from build123d import *

# Parameters (mm, degrees)
F1_DEPTH = 12.7
F2_R     = 1.27


with BuildPart() as f1:
    # F0 (on Top) → F1 (new body)
    with BuildSketch(Plane.XY):
        with BuildLine():
            ThreePointArc((-11.2866647297, 31.0098564859), (0, 33), (11.2866647297, 31.0098564859))
            Line((11.2866647297, 31.0098564859), (11.7129790451, 32.1811454409))
            ThreePointArc((11.7129790451, 32.1811454409), (11.6604357653, 33.1734751566), (10.9094104776, 33.8241978919))
            ThreePointArc((10.9094104776, 33.8241978919), (7.8564465257, 34.6607537135), (4.7411554622, 35.2223373001))
            ThreePointArc((4.7411554622, 35.2223373001), (3.167898391, 36.0676691962), (2.54, 37.7396343385))
            Line((2.54, 37.7396343385), (2.54, 39.2591184658))
            Line((2.54, 39.2591184658), (6.35, 39.2591184658))
            ThreePointArc((6.35, 39.2591184658), (7.2480256121, 39.6310928537), (7.62, 40.5291184658))
            Line((7.62, 40.5291184658), (7.62, 42.4341184658))
            Line((7.62, 42.4341184658), (2.54, 42.4341184658))
            Line((2.54, 42.4341184658), (2.54, 44.9741184658))
            Line((2.54, 44.9741184658), (4.318, 44.9741184658))
            ThreePointArc((4.318, 44.9741184658), (5.2160256121, 45.3460928537), (5.588, 46.2441184658))
            Line((5.588, 46.2441184658), (5.588, 46.5616184658))
            Line((5.588, 46.5616184658), (2.9195765878, 49.6191869589))
            ThreePointArc((2.9195765878, 49.6191869589), (2.488257012, 49.9402838921), (1.9627272727, 50.0541184658))
            Line((1.9627272727, 50.0541184658), (0, 50.0541184658))
            Line((0, 50.0541184658), (-1.9627272727, 50.0541184658))
            ThreePointArc((-1.9627272727, 50.0541184658), (-2.488257012, 49.9402838921), (-2.9195765878, 49.6191869589))
            Line((-2.9195765878, 49.6191869589), (-5.588, 46.5616184658))
            Line((-5.588, 46.5616184658), (-5.588, 46.2441184658))
            ThreePointArc((-5.588, 46.2441184658), (-5.2160256121, 45.3460928537), (-4.318, 44.9741184658))
            Line((-4.318, 44.9741184658), (-2.54, 44.9741184658))
            Line((-2.54, 44.9741184658), (-2.54, 42.4341184658))
            Line((-2.54, 42.4341184658), (-7.62, 42.4341184658))
            Line((-7.62, 42.4341184658), (-7.62, 40.5291184658))
            ThreePointArc((-7.62, 40.5291184658), (-7.2480256121, 39.6310928537), (-6.35, 39.2591184658))
            Line((-6.35, 39.2591184658), (-2.54, 39.2591184658))
            Line((-2.54, 39.2591184658), (-2.54, 37.7396343385))
            ThreePointArc((-2.54, 37.7396343385), (-3.167898391, 36.0676691962), (-4.7411554622, 35.2223373001))
            ThreePointArc((-4.7411554622, 35.2223373001), (-7.8564465257, 34.6607537135), (-10.9094104776, 33.8241978919))
            ThreePointArc((-10.9094104776, 33.8241978919), (-11.6604357653, 33.1734751566), (-11.7129790451, 32.1811454409))
            Line((-11.7129790451, 32.1811454409), (-11.2866647297, 31.0098564859))
        make_face()
    extrude(amount=F1_DEPTH)

    # F2
    f2_edges = [f1.edges().sort_by_distance(p)[0] for p in [
        (3.167898, 36.067669, 12.7),
        (-7.856447, 34.660754, 12.7),
        (-5.08, 42.434118, 12.7),
        (5.08, 42.434118, 12.7),
        (4.253788, 48.090403, 12.7),
    ]]
    fillet(f2_edges, radius=F2_R)


solid = f1.part
CAD build for the part. Positions are in the model's coordinates, mm. A direction names the side the tool comes from. Round coordinates to 2 decimals unless told otherwise and drop trailing zeros. Write each loop counter-clockwise with the first axis right and the second up, starting at its lowest first coordinate (ties: lowest second). Pieces come first, ordered by that corner, then holes. Notation, with made-up numbers: M -22.5,-19.5 L 19.5,-19.5 A23 ccw 19.5,13.5 Z; hole C 4.25,-14.75 d7. An arc over 180 degrees is marked long. Use a Markdown table: item, result. Add a question column.
1. Pull direction Y, two halves, no side cores. Call faces 1 (the face through (-2.481, 49.943, 5.635)), 2 (the face through (7.238, 39.621, 6.261)), 3 (the face through (0, 40, 12.7)), 4 (the face through (11.16, 31.72, 12.32)): released by +Y, released by -Y, zero draft, split by the parting line, or undercut.
2. 3-axis set-ups, long thin cutter, end or side, ignore diameter. For faces 5 (the face through (5, 42.434, 6)), 6 (the face through (7.62, 41, 6)), 7 (the face through (-7.81, 34.67, 5.63)): which of +Z, -Z, +X, -X, +Y, -Y reach the whole face in a straight line?
3. Slice it at B-B on y = 42. Give the cut face in (x, z), then the cut area to 3 significant figures.
4. Drill centre lines: probe 1 along X at (y, z) = (46.25, 9.5); probe 2 along Y at (x, z) = (-5, 7); probe 3 along X at (y, z) = (44, 10.5). Where is each one in solid material? Low to high.
5. Slice it at C-C on x = -3.75. Give the number of separate pieces and of enclosed holes in the cut face, then the cut area to 3 significant figures.
6. Flat gauge pins, fed straight in: P1, Ø1.9, axis at y = 43.5, z = 7, coming from the -X side; P2, Ø1.5, axis at x = 4.5, z = 3.5, coming from the +Y side; P3, Ø2, axis at x = -3, z = 4, coming from the -Y side. Where does each tip first touch, or does it go through?
Reply:
| question | item | result |
|---|---|---|
| 1 | face 1 | released by +Y |
| 1 | face 2 | undercut |
| 1 | face 3 | zero draft |
| 1 | face 4 | released by -Y |
| 2 | face 5 | +Z, -Z, +X |
| 2 | face 6 | +Z, -Z, +X, +Y |
| 2 | face 7 | +Z, -Z, -X |
| 3 | outline | M -7.62,0 L 7.62,0 L 7.62,12.39 L 2.54,12.39 L 2.54,12.7 L -2.54,12.7 L -2.54,12.39 L -7.62,12.39 Z |
| 3 | area | 190 mm^2 |
| 4 | probe 1 | x = -5.59 to 5.59 |
| 4 | probe 2 | y = 32.62 to 35.19, 39.26 to 42.43, 45.17 to 47.24 |
| 4 | probe 3 | x = -2.54 to 2.54 |
| 5 | separate pieces | 3 |
| 5 | enclosed holes | 0 |
| 5 | area | 121 mm^2 |
| 6 | P1 | stops at x = -2.54 |
| 6 | P2 | stops at y = 48.67 |
| 6 | P3 | stops at y = 32.76 |
